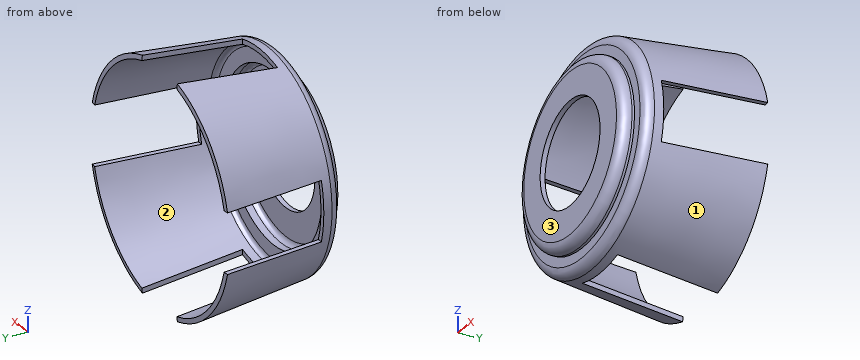
from build123d import *

# Parameters (mm, degrees)
CUT_EXTRUDE1_REACH = 88.028
SKETCH2_W          = 24.54
SKETCH2_H          = 40.87
CIRPATTERN1_COUNT  = 4
CUT_EXTRUDE2_REACH = 87.485
SKETCH3_R          = 21


with BuildPart() as part:
    # Sketch1 → Revolve-Thin1 (revolve)
    with BuildSketch(Plane.XY, mode=Mode.PRIVATE) as revolve_thin1_sk:
        with BuildLine():
            Line((0, 0), (32.5, 0))
            ThreePointArc((32.5, 0), (33.914213562, 0.585786438), (34.5, 2))
            Line((34.5, 2), (34.5, 5))
            Line((34.5, 5), (40.364397089, 5))
            ThreePointArc((40.364397089, 5), (41.702658302, 5.513710349), (42.35344088, 6.790943073))
            Line((42.35344088, 6.790943073), (47, 51))
            Line((47, 51), (48.989043791, 50.790943073))
            Line((48.989043791, 50.790943073), (44.342484671, 6.581886147))
            ThreePointArc((44.342484671, 6.581886147), (43.040919515, 4.027420698), (40.364397089, 3))
            Line((40.364397089, 3), (36.5, 3))
            Line((36.5, 3), (36.5, 2))
            ThreePointArc((36.5, 2), (35.328427125, -0.828427125), (32.5, -2))
            Line((32.5, -2), (0, -2))
            Line((0, -2), (0, 0))
        make_face()
    revolve(revolve_thin1_sk.sketch.rotate(Axis((0, 0, 0), (0, 1, 0)), 90), axis=Axis((0, 0, 0), (0, 1, 0)))

    # Sketch2 → Cut-Extrude1 (cut, up to next)
    with BuildSketch(Plane.XY, mode=Mode.PRIVATE) as cut_extrude1_sk1:
        with Locations((0, 30.565)):
            Rectangle(SKETCH2_W, SKETCH2_H)
    cut_extrude1_tool1 = extrude(cut_extrude1_sk1.sketch, amount=CUT_EXTRUDE1_REACH, mode=Mode.PRIVATE) & part.part
    cut_extrude1 = cut_extrude1_tool1.solids().sort_by_distance((0, 30.565, 0))[0]
    add(cut_extrude1, mode=Mode.SUBTRACT)

    # CirPattern1: Cut-Extrude1 ×4 about axis
    cirpattern1_axis = Axis((0, 0, 0), (0, 1, 0))
    for i in range(1, CIRPATTERN1_COUNT):
        add(cut_extrude1.rotate(cirpattern1_axis, i * 360 / CIRPATTERN1_COUNT), mode=Mode.SUBTRACT)

    # Sketch3 → Cut-Extrude2 (cut, up to next)
    with BuildSketch(Plane.XZ.offset(2), mode=Mode.PRIVATE) as cut_extrude2_sk1:
        with Locations(Location((0, 0, 0), (0, 0, 270))):
            Circle(SKETCH3_R)
    cut_extrude2_tool1 = extrude(cut_extrude2_sk1.sketch, amount=-CUT_EXTRUDE2_REACH, mode=Mode.PRIVATE) & part.part
    add(cut_extrude2_tool1.solids().sort_by_distance((0, -2, 0))[0], mode=Mode.SUBTRACT)


solid = part.part
Can you work these out from the model? Positions are in its coordinate system, mm. Face numbers are marked on the shaded views. Coordinates: 2 decimals unless noted, no trailing zeros. Order: outer loops, then holes, each group sorted by start corner. A loop starts at its lowest first (then second) coordinate and runs counter-clockwise, first axis right, second up. Notation, with made-up numbers: (43.5, 39) - (59.5, 39) arc R19 cw to (59.5, 63) - close; hole circle Ø11 at (69, 12). An arc over 180 degrees is marked (long way). Answer as a JSON object with one key per item and string values. Group by question number.
Q1. I need wall thicknesses on line 1 (X direction, y = 2.7, z = 0); line 2 (Y direction, x = 0, z = 38); line 3 (Z direction, x = 19.5, y = 18). Which ranges of each line are inside material? Lowest first, please. Write a range as from..to.
Q2. Imagine slicing it at C-C (z = 0). Please give me the cut outline in (x, y), and give its area (3 significant figures).
Q3. We'd pull the mould along X, two halves only. Please class the marked faces 1, 2 and 3: +X half, -X half, draft (parallel to the pull), parting line (faces both ways), or undercut.
Q4. Will these pins go through, and if not, where does the flat tip stop? P1, Ø1.5, axis at y = 44, z = 18, coming from the -X side; P2, Ø1.9, axis at x = 2.5, z = 43, coming from the +Y side; P3, Ø5, axis at y = 21, z = -45, coming from the -X side.
Q5. Imagine slicing it at A-A (y = 41.5). Please give me the cut outline in (x, z), and give its area (3 significant figures).
Q6. Imagine slicing it at B-B (x = 0). Please give me the cut outline in (y, z), and give its area (3 significant figures).
Q7. Imagine slicing it at D-D (y = 47.5). Please give me the cut outline in (x, z), and give its area (3 significant figures).
Determined:
{
 "1": {"line 1": "x = -36.5..-34.5, 34.5..36.5", "line 2": "y = 3..5", "line 3": "z = -41.16..-38.92, 38.92..41.16"},
 "2": {"outline": "(-44.72, 10.13) - (-44.34, 6.58) arc R4 ccw to (-40.36, 3) - (-36.5, 3) - (-36.5, 2) arc R4 ccw to (-32.5, -2) - (-21, -2) - (-21, 0) - (-32.5, 0) arc R2 cw to (-34.5, 2) - (-34.5, 5) - (-40.36, 5) arc R2 cw to (-42.35, 6.79) - (-42.7, 10.13) - close; (21, -2) - (32.5, -2) arc R4 ccw to (36.5, 2) - (36.5, 3) - (40.36, 3) arc R4 ccw to (44.34, 6.58) - (44.72, 10.13) - (42.7, 10.13) - (42.35, 6.79) arc R2 cw to (40.36, 5) - (34.5, 5) - (34.5, 2) arc R2 cw to (32.5, 0) - (21, 0) - close", "area": "124 mm2"},
 "3": {"face 1": "parting line", "face 2": "undercut", "face 3": "draft"},
 "4": {"P1": "stops at x = -45.1", "P2": "stops at y = 10.13", "P3": "stops at x = -17.26"},
 "5": {"outline": "(-46.42, -12.27) arc R48.01 ccw to (-12.27, -46.42) - (-12.27, -44.33) arc R46 cw to (-44.33, -12.27) - close; (-46.42, 12.27) - (-44.33, 12.27) arc R46 cw to (-12.27, 44.33) - (-12.27, 46.42) arc R48.01 ccw to start; (12.27, -46.42) arc R48.01 ccw to (46.42, -12.27) - (44.33, -12.27) arc R46 cw to (12.27, -44.33) - close; (12.27, 44.33) arc R46 cw to (44.33, 12.27) - (46.42, 12.27) arc R48.01 ccw to (12.27, 46.42) - close", "area": "394 mm2"},
 "6": {"outline": "(-2, -32.5) arc R4 ccw to (2, -36.5) - (3, -36.5) - (3, -40.36) arc R4 ccw to (6.58, -44.34) - (10.13, -44.72) - (10.13, -42.7) - (6.79, -42.35) arc R2 cw to (5, -40.36) - (5, -34.5) - (2, -34.5) arc R2 cw to (0, -32.5) - (0, -21) - (-2, -21) - close; (-2, 21) - (0, 21) - (0, 32.5) arc R2 cw to (2, 34.5) - (5, 34.5) - (5, 40.36) arc R2 cw to (6.79, 42.35) - (10.13, 42.7) - (10.13, 44.72) - (6.58, 44.34) arc R4 ccw to (3, 40.36) - (3, 36.5) - (2, 36.5) arc R4 ccw to (-2, 32.5) - close", "area": "124 mm2"},
 "7": {"outline": "(-47.07, -12.27) arc R48.64 ccw to (-12.27, -47.07) - (-12.27, -44.99) arc R46.63 cw to (-44.99, -12.27) - close; (-47.07, 12.27) - (-44.99, 12.27) arc R46.63 cw to (-12.27, 44.99) - (-12.27, 47.07) arc R48.64 ccw to start; (12.27, -47.07) arc R48.64 ccw to (47.07, -12.27) - (44.99, -12.27) arc R46.63 cw to (12.27, -44.99) - close; (12.27, 44.99) arc R46.63 cw to (44.99, 12.27) - (47.07, 12.27) arc R48.64 ccw to (12.27, 47.07) - close", "area": "402 mm2"}
}
